Input: part model. Units: mm. Frame: model coordinates. A direction names the side the tool comes from. Round coordinates to 2 decimals unless told otherwise and drop trailing zeros. Order: outer loops, then holes, each group sorted by start corner. A loop starts at its lowest first (then second) coordinate and runs counter-clockwise, first axis right, second up. Notation, with made-up numbers: (60, 30) -> (96, 30) arc R32 ccw to (96, 59) -> close; hole circle Ø7 at (56, 31). An arc over 180 degrees is marked (long way). Use a Markdown table: item, result.
from build123d import *

# Parameters (mm, degrees)
SKETCH1_R           = 21.971
BOSS_EXTRUDE1_DEPTH = 10.16
SKETCH2_W           = 3.175
SKETCH2_H           = 7.239
SKETCH3_R           = 12.5095
BOSS_EXTRUDE2_DEPTH = 5.969
SKETCH4_R           = 3.9751
CUT_EXTRUDE1_DEPTH  = 17.129


with BuildPart() as part:
    # Sketch1 → Boss-Extrude1 (new body)
    with BuildSketch(Plane(origin=(0, 0, 0), x_dir=(1, 0, 0), z_dir=(0, 1, 0))):
        Circle(SKETCH1_R)
    extrude(amount=BOSS_EXTRUDE1_DEPTH)

    # Sketch2 → Cut-Revolve1 (revolve, cut)
    with BuildSketch(Plane.XY):
        with Locations((-20.3835, 5.08)):
            Rectangle(SKETCH2_W, SKETCH2_H)
    revolve(axis=Axis((0, 0, 0), (0, 1, 0)), mode=Mode.SUBTRACT)

    # Sketch3 → Boss-Extrude2 (add)
    with BuildSketch(Plane(origin=(0, 10.16, 0), x_dir=(1, 0, 0), z_dir=(0, 1, 0))):
        Circle(SKETCH3_R)
    extrude(amount=BOSS_EXTRUDE2_DEPTH)

    # Sketch4 → Cut-Extrude1 (cut, through all)
    with BuildSketch(Plane(origin=(0, 16.129, 0), x_dir=(1, 0, 0), z_dir=(0, 1, 0))):
        Circle(SKETCH4_R)
    extrude(amount=-CUT_EXTRUDE1_DEPTH, mode=Mode.SUBTRACT)


solid = part.part
1) Cut plane A-A on z = 0. Return loops of the section in (x, y), and give its area (3 significant figures).
Results found:
| item | result |
|---|---|
| outline | (-21.97, 0) -> (-3.98, 0) -> (-3.98, 16.13) -> (-12.51, 16.13) -> (-12.51, 10.16) -> (-21.97, 10.16) -> (-21.97, 8.7) -> (-18.8, 8.7) -> (-18.8, 1.46) -> (-21.97, 1.46) -> close; (3.98, 0) -> (21.97, 0) -> (21.97, 1.46) -> (18.8, 1.46) -> (18.8, 8.7) -> (21.97, 8.7) -> (21.97, 10.16) -> (12.51, 10.16) -> (12.51, 16.13) -> (3.98, 16.13) -> close |
| area | 422 mm² |
2) Set-up query: faces 1 (the cylindrical face through (2.447, 5.131, 18.636)), 2 (the flat face through (-3, 16.129, -3)). Return all of +Z, -Z, +X, -X, +Y, -Y with unobstructed straight access to the full face (end or side cutting, diameter ignored); none if empty.
Results found:
| item | result |
|---|---|
| face 1 | none |
| face 2 | +Z, -Z, +X, -X, +Y |
3) Cut plane D-D on z = -5. Return loops of the section in (x, y), and give its area (3 significant figures).
Results found:
| item | result |
|---|---|
| outline | (-21.39, 0) -> (21.39, 0) -> (21.39, 1.46) -> (18.12, 1.46) -> (18.12, 8.7) -> (21.39, 8.7) -> (21.39, 10.16) -> (11.47, 10.16) -> (11.47, 16.13) -> (-11.47, 16.13) -> (-11.47, 10.16) -> (-21.39, 10.16) -> (-21.39, 8.7) -> (-18.12, 8.7) -> (-18.12, 1.46) -> (-21.39, 1.46) -> close |
| area | 524 mm² |
4) Cut plane B-B on x = 0. Return loops of the section in (y, z), and give its area (3 significant figures).
Results found:
| item | result |
|---|---|
| outline | (0, -21.97) -> (1.46, -21.97) -> (1.46, -18.8) -> (8.7, -18.8) -> (8.7, -21.97) -> (10.16, -21.97) -> (10.16, -12.51) -> (16.13, -12.51) -> (16.13, -3.98) -> (0, -3.98) -> close; (0, 3.98) -> (16.13, 3.98) -> (16.13, 12.51) -> (10.16, 12.51) -> (10.16, 21.97) -> (8.7, 21.97) -> (8.7, 18.8) -> (1.46, 18.8) -> (1.46, 21.97) -> (0, 21.97) -> close |
| area | 422 mm² |
5) Pin query (flat end, axial travel): pin 1 Ø3 at (y, z) = (3.5, -10) entering from +X; pin 2 Ø3 at (x, y) = (12, 9.5) entering from +Z; pin 3 Ø1.5 at (x, y) = (17, 8.5) entering from -Z. Return the tip coordinate at first contact, or that it passes through.
Results found:
| item | result |
|---|---|
| pin 1 | stops at x = 16.76 |
| pin 2 | stops at z = 19.3 |
| pin 3 | stops at z = -14.76 |
6) Pull-direction query (Y, two-part tool) for faces 3 (the cylindrical face through (-1.628, 13.103, -12.403)), 4 (the flat face through (9, 10.16, 9)), 5 (the flat face through (-16.2, 8.7, 9.9)); classes: +Y half, -Y half, draft (parallel to the pull), parting line (faces both ways), or undercut.
Results found:
| item | result |
|---|---|
| face 3 | draft |
| face 4 | +Y half |
| face 5 | undercut |
7) Line query: L1, parallel to X at y = 9.5, z = 0; L2, parallel to X at y = 10.25, z = 0. Output: solid intervals per line, ascending. Write a range as [from, to].
Results found:
| item | result |
|---|---|
| L1 | x = [-21.97, -3.98], [3.98, 21.97] |
| L2 | x = [-12.51, -3.98], [3.98, 12.51] |
8) Cut plane C-C on y = 12. Return loops of the section in (x, z), and give its area (3 significant figures).
Results found:
| item | result |
|---|---|
| outline | circle Ø25.02 at (0, 0); hole circle Ø7.95 at (0, 0) |
| area | 442 mm² |
